For this review, use the dimensioned drawing (mm, ordinates from the lowest corner) and the shaded views. A direction names the side the tool comes from. Coordinates: 2 decimals unless noted, no trailing zeros. Loops run counter-clockwise (first coordinate to the right, second up) from the corner with the lowest first, then second, coordinate; pieces in that order, holes last. Notation, with made-up numbers: (54, 67) - (93, 67) arc R28 ccw to (93, 96) - close; hole circle Ø1 at (20.5, 8.25). An arc over 180 degrees is marked (long way). Answer in a Markdown table with one row per item. Add a question column.
(1) To check wall thickness, follow L1, parallel to Y at x = 9.25, z = 1.5; L2, parallel to Z at x = 17.25, y = 17.25; L3, parallel to X at y = 14.25, z = 0.5 (1 decimal). State the ranges of each line that lie inside material, in increasing order. Write a range as [from, to].
(2) Clearance check with flat-ended pins moving along their axes: pin 1 (1 mm diameter, centred on x = 11, z = 0.5, fed in from +Y); pin 2 (0.6 mm diameter, centred on y = 2.5, z = 0.5, fed in from +X); pin 3 (0.6 mm diameter, centred on y = 2.5, z = 0.5, fed in from -X); pin 4 (2 mm diameter, centred on x = 14.5, y = 2.5, fed in from -Z). State where each tip first meets the part, or that it passes through.
(3) We need section D-D, the plane y = 1.75. Write out the cut boundary in (x, z).
(4) The part is to be moulded in two halves that separate along X. For the marked faces 1, 2, 3 and 4, say which applies: released by +X, released by -X, zero draft, split by the parting line, or undercut.
(5) We need section B-B, the plane y = 9.5. Write out the cut boundary in (x, z), plus the area to 3 significant figures.
(6) We need section A-A, the plane z = 1.25. Write out the cut boundary in (x, y), plus the area to 3 significant figures.
(7) For the marked faces 5 and 6, list the 3-axis set-ups (+Z, -Z, +X, -X, +Y, -Y) from which the entire face can be reached by the end or side of a thin tool; tool diameter is ignored.
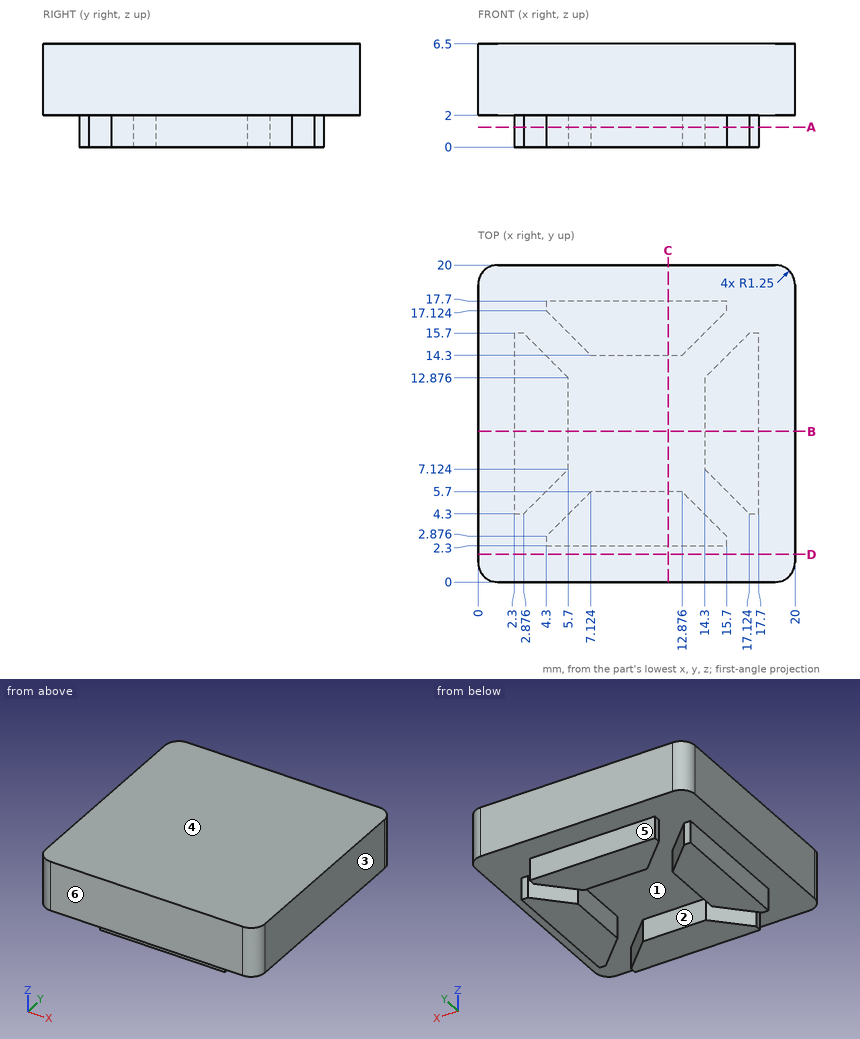
Responses:
| question | item | result |
|---|---|---|
| 1 | L1 | y = [2.3, 5.7], [14.3, 17.7] |
| 1 | L2 | z = [2, 6.5] |
| 1 | L3 | x = [2.3, 4.3], [15.7, 17.7] |
| 2 | pin 1 | stops at y = 17.7 |
| 2 | pin 2 | stops at x = 15.7 |
| 2 | pin 3 | stops at x = 4.3 |
| 2 | pin 4 | stops at z = 0 |
| 3 | outline | (0, 2) - (20, 2) - (20, 6.5) - (0, 6.5) - close |
| 4 | face 1 | undercut |
| 4 | face 2 | undercut |
| 4 | face 3 | released by +X |
| 4 | face 4 | zero draft |
| 5 | outline | (0, 2) - (2.3, 2) - (2.3, 0) - (5.7, 0) - (5.7, 2) - (14.3, 2) - (14.3, 0) - (17.7, 0) - (17.7, 2) - (20, 2) - (20, 6.5) - (0, 6.5) - close |
| 5 | area | 104 mm2 |
| 6 | outline | (2.3, 4.3) - (2.88, 4.3) - (5.7, 7.12) - (5.7, 12.88) - (2.88, 15.7) - (2.3, 15.7) - close; (4.3, 2.3) - (15.7, 2.3) - (15.7, 2.88) - (12.88, 5.7) - (7.12, 5.7) - (4.3, 2.88) - close; (4.3, 17.12) - (7.12, 14.3) - (12.88, 14.3) - (15.7, 17.12) - (15.7, 17.7) - (4.3, 17.7) - close; (14.3, 7.12) - (17.12, 4.3) - (17.7, 4.3) - (17.7, 15.7) - (17.12, 15.7) - (14.3, 12.88) - close |
| 6 | area | 123 mm2 |
| 7 | face 5 | -Z, +X, -X, +Y |
| 7 | face 6 | +Z, -Z, +X, -X, -Y |
